Could you check a few things on this model? Use its own coordinates, in mm. Face numbers are marked on the shaded views. A direction names the side the tool comes from. Give positions to 0.01 mm unless a question says otherwise; leave off trailing zeros. Write each loop counter-clockwise with the first axis right and the second up, starting at its lowest first coordinate (ties: lowest second). Pieces come first, ordered by that corner, then holes. Notation, with made-up numbers: (83.5, -16) - (120.5, -16) arc R35 cw to (120.5, 22) - close; hole circle Ø10 at (1, 58.5). An arc over 180 degrees is marked (long way). Answer in a Markdown table with one row per item.
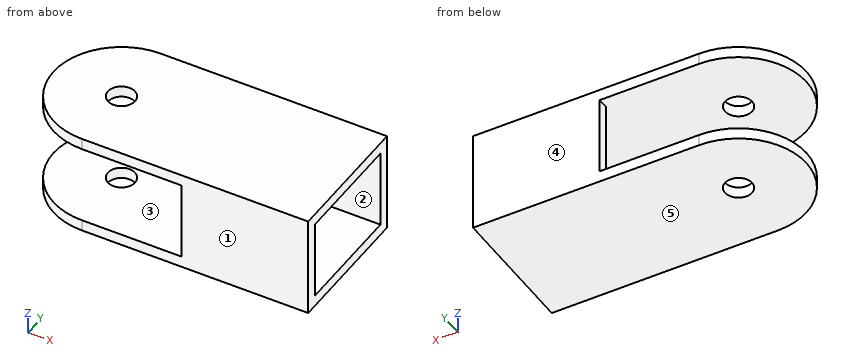
from build123d import *

# Parameters (mm, degrees)
DODANIE_WYCI_GNI_CIE1_DEPTH = 5
SZKIC2_W                    = 56
SZKIC2_H                    = 35
DODANIE_WYCI_GNI_CIE2_DEPTH = 5
SZKIC3_R                    = 6
WYTNIJ_WYCI_GNI_CIE1_DEPTH  = 97.566039579


with BuildPart() as part:
    # Szkic1 → Dodanie-wyci_gni_cie1 (new body)
    with BuildSketch(Plane.XY):
        with BuildLine():
            Line((-50, -30), (50, -30))
            Line((50, -30), (50, 30))
            Line((50, 30), (-50, 30))
            ThreePointArc((-50, 30), (-80, 0), (-50, -30))
        make_face()
    extrude(amount=DODANIE_WYCI_GNI_CIE1_DEPTH)


with BuildPart() as body_2:
    # Lustro2: mirrored copy
    add(part.part.mirror(Plane.XY.offset(22.5)))


with BuildPart() as part_1:
    add(part.part)

    add(body_2.part)  # Dodanie-wyci_gni_cie2 merges body 2
    # Szkic2 → Dodanie-wyci_gni_cie2 (add)
    with BuildSketch(Plane(origin=(0, 30, 0), x_dir=(1, 0, 0), z_dir=(0, 1, 0))):
        with Locations((22, -22.5)):
            Rectangle(SZKIC2_W, SZKIC2_H)
    dodanie_wyci_gni_cie2 = extrude(amount=-DODANIE_WYCI_GNI_CIE2_DEPTH)

    # Lustro3: Dodanie-wyci_gni_cie2 across plane
    add(dodanie_wyci_gni_cie2.mirror(Plane.ZX))

    # Szkic3 → Wytnij-wyci_gni_cie1 (cut, through all)
    with BuildSketch(Plane.XY.offset(45)):
        with Locations((-50, 0)):
            Circle(SZKIC3_R)
    extrude(amount=-WYTNIJ_WYCI_GNI_CIE1_DEPTH, mode=Mode.SUBTRACT)


solid = part_1.part
1) Imagine slicing it at A-A (y = 0). List the corners of the cut face in (x, z) for me.
Check values:
| item | result |
|---|---|
| outline | (-80, 0) - (-56, 0) - (-56, 5) - (-80, 5) - close; (-80, 40) - (-56, 40) - (-56, 45) - (-80, 45) - close; (-44, 0) - (50, 0) - (50, 5) - (-44, 5) - close; (-44, 40) - (50, 40) - (50, 45) - (-44, 45) - close |
2) Imagine slicing it at D-D (x = 35.5). List the corners of the cut face in (y, z) for me.
Check values:
| item | result |
|---|---|
| outline | (-30, 0) - (30, 0) - (30, 45) - (-30, 45) - close; hole (-25, 5) - (25, 5) - (25, 40) - (-25, 40) - close |
3) If I drill on line 1 (Z direction, x = -58.5, y = -20); line 2 (Y direction, x = -50, z = 2.1); line 3 (Y direction, x = 20.5, z = 15), over which ranges is the centre line in solid material (lowest first)?
Check values:
| item | result |
|---|---|
| line 1 | z = 0 to 5, 40 to 45 |
| line 2 | y = -30 to -6, 6 to 30 |
| line 3 | y = -30 to -25, 25 to 30 |
4) Imagine slicing it at B-B (x = -13). List the corners of the cut face in (y, z) for me.
Check values:
| item | result |
|---|---|
| outline | (-30, 0) - (30, 0) - (30, 5) - (-30, 5) - close; (-30, 40) - (30, 40) - (30, 45) - (-30, 45) - close |
5) On a 3-axis mill with a long thin cutter (end or side, diameter ignored), from which of +Z, -Z, +X, -X, +Y, -Y can I reach the whole of each face in a straight line? I mean the marked faces 1 and 2. Say none if no direction works.
Check values:
| item | result |
|---|---|
| face 1 | +Z, -Z, +X, -X, -Y |
| face 2 | +X, -X |
6) Will these pins go through, and if not, where does the flat tip stop? P1, Ø7, axis at x = -50, y = 0, coming from the +Z side; P2, Ø5.5, axis at y = 27.5, z = 21.5, coming from the -X side; P3, Ø12, axis at y = 16.5, z = 8.5, coming from the -X side.
Check values:
| item | result |
|---|---|
| P1 | passes through |
| P2 | stops at x = -6 |
| P3 | stops at x = -77.66 |
7) Imagine slicing it at C-C (z = 35.5). List the corners of the cut face in (x, y) for me, then the cut area to 3 significant figures.
Check values:
| item | result |
|---|---|
| outline | (-6, -30) - (50, -30) - (50, -25) - (-6, -25) - close; (-6, 25) - (50, 25) - (50, 30) - (-6, 30) - close |
| area | 560 mm2 |
8) We'd pull the mould along Z, two halves only. Please class the marked faces 3, 4 and 5: +Z half, -Z half, draft (parallel to the pull), parting line (faces both ways), or undercut.
Check values:
| item | result |
|---|---|
| face 3 | undercut |
| face 4 | draft |
| face 5 | -Z half |
